Autodesk Inventor part; units mm, degrees
ref_plane "YZ Plane" through (0, 0, 0) normal (1, 0, 0) x (0, 1, 0)
ref_plane "XZ Plane" through (0, 0, 0) normal (0, 1, 0) x (-1, 0, 0)
ref_plane "XY Plane" through (0, 0, 0) normal (0, 0, 1) x (1, 0, 0)
sketch "Sketch1" plane through (0, 0, 0) normal (0, 0, 1) x (1, 0, 0)
  circle A0 centre (0, 0) radius 6.35
  dimension "d0" = 12.7
extrude "Extrusion1" add sketch "Sketch1" along normal blind 304.8
sketch "Sketch2" plane through (0, 0, 304.8) normal (0, 0, 1) x (1, 0, 0)
  circle A0 centre (0, 0) radius 6.35
  circle A1 centre (0, 0) radius 3.429
  circle A2 centre (0, 0) radius 6.35
  dimension "d3" = 6.858
extrude "Extrusion2" cut sketch "Sketch2" against normal blind 25.4
sketch "Sketch3" plane through (0, 0, 0) normal (0, 0, -1) x (-1, 0, 0)
  circle A0 centre (0, 0) radius 6.35
  arc A1 (1.5875, 6.1484) -> (-1.5875, 6.1484) centre (0, 0) ccw
  line L0 (-1.5875, 6.1484) -> (-1.5875, 4.7625)
  line L1 (-1.5875, 4.7625) -> (1.5875, 4.7625)
  line L2 (1.5875, 4.7625) -> (1.5875, 6.1484)
  line L3 (0, 6.35) -> (1.0636, 6.35) construction
  dimension "d6" = 3.175
  dimension "d7" = 1.5875
extrude "Extrusion3" cut sketch "Sketch3" against normal blind 203.2 contours L2 L1 L0 A0 picked at (0.1781, 5.2842)
properties part number "ShooterAxle" material "Steel"
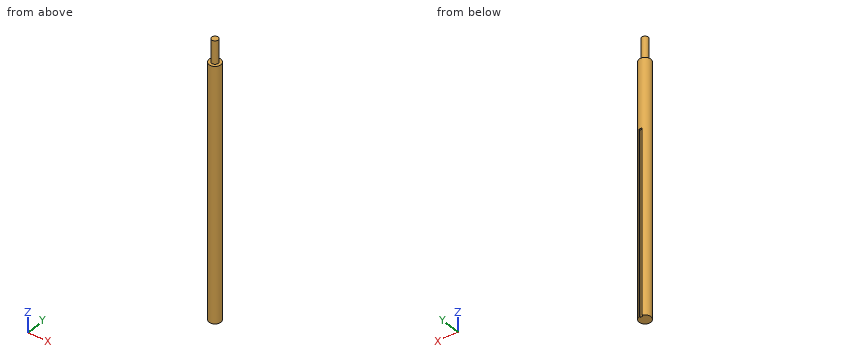
Verification items for the finished model (mm, model axes). Round coordinates to 2 decimals unless told otherwise and drop trailing zeros. Loops run counter-clockwise (first coordinate to the right, second up) from the corner with the lowest first, then second, coordinate; pieces in that order, holes last. Notation, with made-up numbers: (19, 12.25) - (47, 12.25) arc R9 cw to (47, 20.25) - close; hole circle Ø8 at (-32.5, -2.5). An arc over 180 degrees is marked (long way). Use one line per item in the form item = value.
1. Section check B-B on z = 245.5. Record the cut outline in (x, y), and give its area (3 significant figures).
A:
outline = circle Ø12.7 at (0, 0)
area = 127 mm²
2. Scan lines: probe 1 along Z at (x, y) = (1.25, -5.25); probe 2 along X at (y, z) = (-0.5, 40); probe 3 along Y at (x, z) = (-0.5, 177.5). Record each from-to range of solid material in increasing order.
A:
probe_1 = 0 to 279.4
probe_2 = -6.33 to 6.33
probe_3 = -6.33 to 4.76
3. Section check A-A on y = 0. Record the cut outline in (x, z), and give its area (3 significant figures).
A:
outline = (-6.35, 0) - (6.35, 0) - (6.35, 279.4) - (3.43, 279.4) - (3.43, 304.8) - (-3.43, 304.8) - (-3.43, 279.4) - (-6.35, 279.4) - close
area = 3,720 mm²
4. Gauge pin test, flat ends, axial feed: pin 1 Ø1 at (y, z) = (4.5, 187.5) entering from +X; pin 2 Ø1 at (y, z) = (0.5, 80.5) entering from -X; pin 3 Ø2 at (x, z) = (-1.5, 51) entering from +Y; pin 4 Ø1.1 at (y, z) = (6, 149) entering from -X. Record the tip position at first contact, or that the pin passes through.
A:
pin_1 = 4.93
pin_2 = -6.35
pin_3 = 6.15
pin_4 = -3.26
5. Section check C-C on z = 130. Record the cut outline in (x, y).
A:
outline = (-1.59, 4.76) - (-1.59, 6.15) arc R6.35 ccw (long way) to (1.59, 6.15) - (1.59, 4.76) - close
